Geometry: final body of the model. Coordinates: model frame, mm. A direction names the side the tool comes from. Round coordinates to 2 decimals unless told otherwise and drop trailing zeros. Order: outer loops, then holes, each group sorted by start corner. A loop starts at its lowest first (then second) coordinate and runs counter-clockwise, first axis right, second up. Notation, with made-up numbers: M 67.25,79.5 L 111.25,79.5 A8 ccw 111.25,83.5 Z; hole C 44.25,6 d10. An arc over 180 degrees is marked long. Return JSON: item names as keys, results as strings. Group by question number.
Q1. Ray query, probe 1 along Z at (x, y) = (15, -1.75); probe 2 along Z at (x, y) = (48.5, -9.5). Return the intervals inside material, ascending.
Q2. Access query for faces 1 (the face through (-39.26, -6.16, 7.17)), 2 (the face through (39.26, -6.16, -7.17)), 3 (the face through (-1, -12.5, 0)). Directions: +Z, -Z, +X, -X, +Y, -Y. A direction counts if a zero-diameter tool reaches every point of the face in a straight line with its end or side. Return the directions, or none.
Q3. Cut plane C-C on x = 32.5. Output: boundary loops of the cut face in (y, z).
Q4. Cut plane A-A on y = -3.25. Output: boundary loops of the cut face in (x, z).
Q5. Contact query for flat-ended pins moving along their axis: pin 1 (3 mm diameter, centred on x = 26, y = -2.5, fed in from +Z); pin 2 (6 mm diameter, centred on x = 8.5, y = -6, fed in from -Z); pin 3 (1.5 mm diameter, centred on x = 46.5, y = -4.5, fed in from +Z). Output: stop coordinate, or through.
Q6. Cut plane B-B on x = -19. Output: boundary loops of the cut face in (y, z).
```python
from build123d import *

# Parameters (mm, degrees)
F1_DEPTH = 12.5


with BuildPart() as f1:
    # F0 (on Front) → F1 (new body)
    with BuildSketch(Plane.XZ):
        with BuildLine():
            Line((28.5, 6.25), (0, 6.25))
            Line((0, 6.25), (-28.5, 6.25))
            ThreePointArc((-28.5, 6.25), (-39.412292, 7.194524), (-50, 10))
            Line((-50, 10), (-100, 10))
            Line((-100, 10), (-100, 0))
            Line((-100, 0), (-100, -10))
            Line((-100, -10), (-50, -10))
            ThreePointArc((-50, -10), (-39.412292, -7.194524), (-28.5, -6.25))
            Line((-28.5, -6.25), (0, -6.25))
            Line((0, -6.25), (28.5, -6.25))
            ThreePointArc((28.5, -6.25), (39.412292, -7.194524), (50, -10))
            Line((50, -10), (100, -10))
            Line((100, -10), (100, 0))
            Line((100, 0), (100, 10))
            Line((100, 10), (50, 10))
            ThreePointArc((50, 10), (39.412292, 7.194524), (28.5, 6.25))
        make_face()
    extrude(amount=F1_DEPTH)


solid = f1.part
```
Result sheet:
{
 "1": {"probe 1": "z = -6.25 to 6.25", "probe 2": "z = -9.48 to 9.48"},
 "2": {"face 1": "+Z, +Y, -Y", "face 2": "-Z, +Y, -Y", "face 3": "+Z, -Z, +X, -X, -Y"},
 "3": {"outline": "M -12.5,-6.38 L 0,-6.38 L 0,6.38 L -12.5,6.38 Z"},
 "4": {"outline": "M -100,-10 L -50,-10 A63.51 cw -28.5,-6.25 L 28.5,-6.25 A63.51 cw 50,-10 L 100,-10 L 100,10 L 50,10 A63.51 cw 28.5,6.25 L -28.5,6.25 A63.51 cw -50,10 L -100,10 Z"},
 "5": {"pin 1": "stops at z = 6.25", "pin 2": "stops at z = -6.25", "pin 3": "stops at z = 9.08"},
 "6": {"outline": "M -12.5,-6.25 L 0,-6.25 L 0,6.25 L -12.5,6.25 Z"}
}
